Geometry: final body of the model. Coordinates: model frame, mm. Face numbers are marked on the shaded views. Give positions to 0.01 mm unless a question says otherwise; leave off trailing zeros. Loops run counter-clockwise (first coordinate to the right, second up) from the corner with the lowest first, then second, coordinate; pieces in that order, holes last. Notation, with made-up numbers: M -35,2 L -13,2 A10 ccw -13,7 Z; hole C 24,62 d4. An arc over 180 degrees is marked long. Put each result on its own line as item: value.
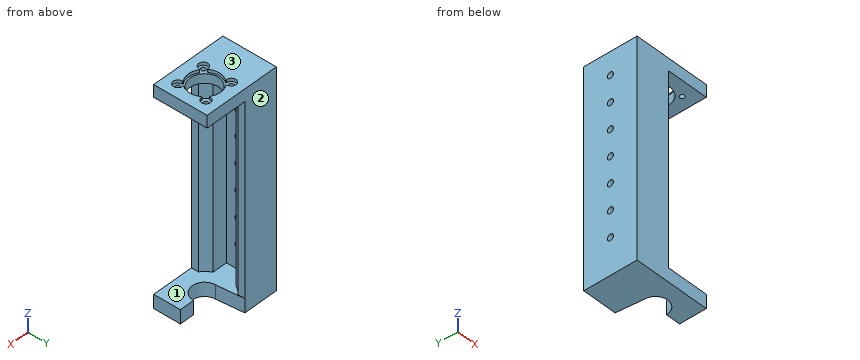
```python
from build123d import *

# Parameters (mm, degrees)
SKETCH1_W           = 50
SKETCH1_H           = 35
SKETCH1_R           = 9.5
SKETCH1_R_2         = 1.5
BOSS_EXTRUDE3_DEPTH = 6
SKETCH4_W           = 50
SKETCH4_H           = 35
BOSS_EXTRUDE5_DEPTH = 2
BOSS_EXTRUDE6_DEPTH = 124
SKETCH9_R           = 2
CUT_EXTRUDE1_DEPTH  = 115
BOSS_EXTRUDE7_DEPTH = 9


with BuildPart() as part:
    # Sketch1 → Boss-Extrude3 (new body)
    with BuildSketch(Plane.XY):
        with Locations((25, 17.5)):
            Rectangle(SKETCH1_W, SKETCH1_H)
        with Locations((32.5, 17.5)):
            Circle(SKETCH1_R, mode=Mode.SUBTRACT)
        with Locations((41.692388155, 26.692388155)):
            Circle(SKETCH1_R_2, mode=Mode.SUBTRACT)
        with Locations((41.692388155, 8.307611845)):
            Circle(SKETCH1_R_2, mode=Mode.SUBTRACT)
        with Locations((23.307611845, 8.307611845)):
            Circle(SKETCH1_R_2, mode=Mode.SUBTRACT)
        with Locations((23.307611845, 26.692388155)):
            Circle(SKETCH1_R_2, mode=Mode.SUBTRACT)
    extrude(amount=BOSS_EXTRUDE3_DEPTH)

    # Sketch4 → Boss-Extrude5 (add)
    with BuildSketch(Plane.XY.offset(6)):
        with Locations((25, 17.5)):
            Rectangle(SKETCH4_W, SKETCH4_H)
        with BuildLine():
            ThreePointArc((26.299419693, 26.47083501), (21.186291501, 28.813708499), (23.52916499, 23.700580307))
            ThreePointArc((23.52916499, 23.700580307), (23.763454109, 23.57743344), (23.755822455, 23.312861521))
            ThreePointArc((23.755822455, 23.312861521), (22, 17.5), (23.755822455, 11.687138479))
            ThreePointArc((23.755822455, 11.687138479), (23.763454109, 11.42256656), (23.52916499, 11.299419693))
            ThreePointArc((23.52916499, 11.299419693), (21.186291501, 6.186291501), (26.299419693, 8.52916499))
            ThreePointArc((26.299419693, 8.52916499), (26.42256656, 8.763454109), (26.687138479, 8.755822455))
            ThreePointArc((26.687138479, 8.755822455), (32.5, 7), (38.312861521, 8.755822455))
            ThreePointArc((38.312861521, 8.755822455), (38.57743344, 8.763454109), (38.700580307, 8.52916499))
            ThreePointArc((38.700580307, 8.52916499), (43.813708499, 6.186291501), (41.47083501, 11.299419693))
            ThreePointArc((41.47083501, 11.299419693), (41.236545891, 11.42256656), (41.244177545, 11.687138479))
            ThreePointArc((41.244177545, 11.687138479), (43, 17.5), (41.244177545, 23.312861521))
            ThreePointArc((41.244177545, 23.312861521), (41.236545891, 23.57743344), (41.47083501, 23.700580307))
            ThreePointArc((41.47083501, 23.700580307), (43.813708499, 28.813708499), (38.700580307, 26.47083501))
            ThreePointArc((38.700580307, 26.47083501), (38.57743344, 26.236545891), (38.312861521, 26.244177545))
            ThreePointArc((38.312861521, 26.244177545), (32.5, 28), (26.687138479, 26.244177545))
            ThreePointArc((26.687138479, 26.244177545), (26.42256656, 26.236545891), (26.299419693, 26.47083501))
        make_face(mode=Mode.SUBTRACT)
    extrude(amount=BOSS_EXTRUDE5_DEPTH)

    # Sketch8 → Boss-Extrude6 (add)
    with BuildSketch(Plane(origin=(0, 0, 0), x_dir=(-1, 0, 0), z_dir=(0, 0, -1))):
        with BuildLine():
            Line((-8.5, 35), (-22.740329685, 35))
            Line((-22.740329685, 35), (-22.740329685, 30.367452558))
            ThreePointArc((-22.740329685, 30.367452558), (-20.171344576, 27.9320063), (-18.194683381, 24.99535966))
            Line((-18.194683381, 24.99535966), (-18.194683381, 25))
            Line((-18.194683381, 25), (-8.5, 25))
            Line((-8.5, 25), (-8.5, 10.000000197))
            Line((-8.5, 10.000000197), (-18.197115572, 10.000000197))
            ThreePointArc((-18.197115572, 10.000000197), (-20.17303677, 7.065994176), (-22.740329685, 4.632547442))
            Line((-22.740329685, 4.632547442), (-22.740329685, 0))
            Line((-22.740329685, 0), (-8.5, 0))
            Line((-8.5, 0), (0, 0))
            Line((0, 0), (0, 10.000000197))
            Line((0, 10.000000197), (0, 25))
            Line((0, 25), (0, 35))
            Line((0, 35), (-8.5, 35))
        make_face()
    extrude(amount=BOSS_EXTRUDE6_DEPTH)

    # Sketch9 → Cut-Extrude1 (cut)
    with BuildSketch(Plane.ZY):
        with Locations((-7, 17.5)):
            Circle(SKETCH9_R)
        with Locations((-24, 17.5)):
            Circle(SKETCH9_R)
        with Locations((-41, 17.5)):
            Circle(SKETCH9_R)
        with Locations((-58, 17.5)):
            Circle(SKETCH9_R)
        with Locations((-75, 17.5)):
            Circle(SKETCH9_R)
        with Locations((-92, 17.5)):
            Circle(SKETCH9_R)
        with Locations((-109, 17.5)):
            Circle(SKETCH9_R)
    extrude(amount=-CUT_EXTRUDE1_DEPTH, mode=Mode.SUBTRACT)

    # Sketch12 → Boss-Extrude7 (add)
    with BuildSketch(Plane(origin=(0, 0, -124), x_dir=(-1, 0, 0), z_dir=(0, 0, -1))):
        with BuildLine():
            Line((-24.5, 17.5), (-22.740329685, 35))
            Line((-22.740329685, 35), (0, 35))
            Line((0, 35), (0, 0))
            Line((0, 0), (-50, 0))
            Line((-50, 0), (-50, 17.5))
            Line((-50, 17.5), (-40.5, 17.5))
            ThreePointArc((-40.5, 17.5), (-32.5, 9.5), (-24.5, 17.5))
        make_face()
    extrude(amount=BOSS_EXTRUDE7_DEPTH)


solid = part.part
```
Item 1: Mould query, pull axis Y, two halves, no side actions, for the marked faces 1, 2 and 3. Classes: pulls with the +Y half, pulls with the -Y half, needs draft (parallel to the pull), parting line crosses it, or undercut.
Output values:
face 1: undercut
face 2: pulls with the +Y half
face 3: needs draft
Item 2: Section B-B on x = 16. Output: boundary loops of the cut face in (y, z), then the cut area to 4 significant figures.
Output values:
outline: M 0,-133 L 35,-133 L 35,8 L 0,8 Z; hole M 10,-124 L 25,-124 L 25,0 L 10,0 Z
area: 3,075 mm²
Item 3: Section D-D on x = 46. Output: boundary loops of the cut face in (y, z), then the cut area to 4 significant figures.
Output values:
outline: M 0,-133 L 17.5,-133 L 17.5,-124 L 0,-124 Z; M 0,0 L 35,0 L 35,8 L 0,8 Z
area: 437.5 mm²
Item 4: Pin query (flat end, axial travel): pin 1 Ø2.5 at (y, z) = (17.5, -75) entering from -X; pin 2 Ø1 at (y, z) = (24, -10.5) entering from -X; pin 3 Ø4.5 at (y, z) = (17.5, -109) entering from +X; pin 4 Ø3.5 at (x, y) = (41.69, 8.31) entering from +Z. Return the tip coordinate at first contact, or that it passes through.
Output values:
pin 1: through
pin 2: x = 0
pin 3: x = 8.5
pin 4: z = 6
Item 5: Section C-C on x = 32.5. Output: boundary loops of the cut face in (y, z), then the cut area to 4 significant figures.
Output values:
outline: M 0,-133 L 9.5,-133 L 9.5,-124 L 0,-124 Z; M 0,0 L 8,0 L 8,6 L 7,6 L 7,8 L 0,8 Z; M 27,0 L 35,0 L 35,8 L 28,8 L 28,6 L 27,6 Z
area: 209.5 mm²
Item 6: Line query: probe 1 along Y at (x, z) = (2, -24); probe 2 along Y at (x, z) = (9, -106); probe 3 along Z at (x, y) = (34, 27). Output: solid intervals per line, ascending. Write a range as [from, to].
Output values:
probe 1: [0, 15.5], [19.5, 35]
probe 2: [0, 10], [25, 35]
probe 3: [0, 6]
